```python
from build123d import *

# Parameters (mm, degrees)
F0_R     = 12.7
F1_DEPTH = 12.7
F2_D     = 9.525


with BuildPart() as f1:
    # F0 (on Front) → F1 (new body)
    with BuildSketch(Plane.XZ):
        with BuildLine():
            Line((-339.485507, -10.16), (-16.114493, -10.16))
            ThreePointArc((-16.114493, -10.16), (19.05, 0), (-16.114493, 10.16))
            Line((-16.114493, 10.16), (-339.485507, 10.16))
            ThreePointArc((-339.485507, 10.16), (-374.65, 0), (-339.485507, -10.16))
        make_face()
        with Locations((-355.6, 0)):
            Circle(F0_R, mode=Mode.SUBTRACT)
        Circle(F0_R, mode=Mode.SUBTRACT)
    extrude(amount=F1_DEPTH)

    # F2 (through all)
    with Locations(Plane(origin=(0, 0, 0), x_dir=(1, 0, 0), z_dir=(0, 1, 0))):
        with Locations((-323.85, 0), (-299.72, 0), (-275.59, 0), (-251.46, 0), (-227.33, 0), (-203.2, 0), (-179.07, 0), (-154.94, 0), (-130.81, 0), (-106.68, 0), (-82.55, 0), (-58.42, 0), (-34.29, 0)):
            Hole(F2_D / 2)


solid = f1.part
```
Can you work these out from the model? Positions are in its coordinate system, mm. A direction names the side the tool comes from. Coordinates: 2 decimals unless noted, no trailing zeros. Loops run counter-clockwise (first coordinate to the right, second up) from the corner with the lowest first, then second, coordinate; pieces in that order, holes last.
Item 1: Suppose I cut it at A-A (x = -34.29). Please give me the cut outline in (y, z), then the cut area to 3 significant figures.
Answers below:
outline: (-12.7, -10.16) - (0, -10.16) - (0, -4.76) - (-12.7, -4.76) - close; (-12.7, 4.76) - (0, 4.76) - (0, 10.16) - (-12.7, 10.16) - close
area: 137 mm2
Item 2: Suppose I cut it at B-B (y = -4.75). State how many separate pieces and enclosed holes the cut face has, then the cut area to 3 significant figures.
Answers below:
separate pieces: 1
enclosed holes: 15
area: 6,830 mm2
Item 3: Which directions (+Z, -Z, +X, -X, +Y, -Y) give clear straight access to the entire face, cutting with the end or side of a thin tool? Please do faces 1 (the face through (-174.312, -6.439, -0.209)), 2 (the face through (-180, -6, -10.16)).
Answers below:
face 1: +Y, -Y
face 2: -Z, +Y, -Y
Item 4: If we mould it in two halves opening along Z, with no side actions, what happens to faces 3 (the face through (-231.873, -6.439, -1.431)), 4 (the face through (-176, -6, 10.16)), 5 (the face through (-374.638, -6.261, 0.688))? For each: released by +Z, released by -Z, zero draft, split by the parting line, or undercut.
Answers below:
face 3: undercut
face 4: released by +Z
face 5: split by the parting line
Item 5: Suppose I cut it at C-C (x = -74.5). Please give me the cut outline in (y, z).
Answers below:
outline: (-12.7, -10.16) - (0, -10.16) - (0, 10.16) - (-12.7, 10.16) - close
Item 6: Please list where these lines run through material, in increasing order: L1, parallel to Z at x = -154.94, y = -9; L2, parallel to X at y = -4, z = -6; L3, parallel to X at y = -9.5, z = -8.
Answers below:
L1: z = -10.16 to -4.76, 4.76 to 10.16
L2: x = -373.68 to -366.79, -344.41 to -11.19, 11.19 to 18.08
L3: x = -372.89 to -365.46, -345.74 to -9.86, 9.86 to 17.29
Item 7: I'm going to push flat-ended pins straight in: pin 1 (4 mm diameter, centred on y = -4.5, z = 14, fed in from -X); pin 2 (8.5 mm diameter, centred on x = -154.94, z = 0, fed in from -Y); pin 3 (1 mm diameter, centred on y = -10.5, z = -11.5, fed in from +X); pin 4 (6.5 mm diameter, centred on x = -152.5, y = -4, fed in from -Z). Where does each tip first touch, or does it pass through?
Answers below:
pin 1: stops at x = -370.4
pin 2: passes through
pin 3: stops at x = 15.55
pin 4: stops at z = -10.16
Item 8: Suppose I cut it at D-D (x = -202). Please give me the cut outline in (y, z), then the cut area to 3 significant figures.
Answers below:
outline: (-12.7, -10.16) - (0, -10.16) - (0, -4.61) - (-12.7, -4.61) - close; (-12.7, 4.61) - (0, 4.61) - (0, 10.16) - (-12.7, 10.16) - close
area: 141 mm2
